```python
from build123d import *

# Parameters (mm, degrees)
CUT_EXTRUDE1_START = 7.29361
CUT_EXTRUDE1_DEPTH = 2.477670997


# Read off the part's stored shape, not the designer's step: Split1
with BuildPart() as part:
    # Sketch2 → Revolve1 (revolve)
    with BuildSketch(Plane(origin=(0, 0, 0), x_dir=(0, 0, -1), z_dir=(1, 0, 0)), mode=Mode.PRIVATE) as revolve1_sk:
        with BuildLine():
            Line((-7.89305, 0.79375), (-7.89305, 1.11125))
            ThreePointArc((-7.89305, 1.11125), (-7.36812089, 2.018629974), (-6.575878571, 2.7051))
            Line((-6.575878571, 2.7051), (-6.39445, 2.7051))
            Line((-6.39445, 2.7051), (-6.39445, 1.4224))
            Line((-6.39445, 1.4224), (7.4168, 1.4224))
            Line((7.4168, 1.4224), (7.89305, 0.94615))
            Line((7.89305, 0.94615), (7.89305, 0))
            Line((7.89305, 0), (-6.835338224, 0))
            Line((-6.835338224, 0), (-7.29361, 0.79375))
            Line((-7.29361, 0.79375), (-7.89305, 0.79375))
        make_face()
    revolve(revolve1_sk.sketch.rotate(Axis((0, 0, 7.89305), (0, 0, -1)), 90), axis=Axis((0, 0, 7.89305), (0, 0, -1)))

    # Sketch3 → Cut-Extrude1 (cut, through all)
    with BuildSketch(Plane.XY.offset(CUT_EXTRUDE1_START)):
        Polygon((0, 0.916543552), (-0.79375, 0.458271776), (-0.79375, -0.458271776), (0, -0.916543552), (0.79375, -0.458271776), (0.79375, 0.458271776), align=None)
    extrude(amount=CUT_EXTRUDE1_DEPTH, mode=Mode.SUBTRACT)

    # Cut-Extrude2 cone 1 section (through the dimple's axis) → Cut-Extrude2 (revolve, cut)
    with BuildSketch(Plane(origin=(0, 0, 7.89305), x_dir=(0, -1, 0), z_dir=(1, 0, 0))):
        Polygon((0, 0), (0.916543552, 0), (0, 0.916543552), align=None)
    revolve(axis=Axis((0, 0, 7.89305), (0, 0, -1)), mode=Mode.SUBTRACT)


with BuildPart() as body_2:
    # Split1: the piece on the far side of the plane
    add(part.part)
    split(bisect_by=Plane.XY.offset(6.39445), keep=Keep.BOTTOM)


with BuildPart() as part_1:
    add(part.part)

    # Split1
    split(bisect_by=Plane.XY.offset(6.39445), keep=Keep.TOP)

    add(body_2.part)  # Boss-Extrude1 merges body 2
    # Boss-Extrude1 cone 1 section (through the dimple's axis) → Boss-Extrude1 (revolve)
    with BuildSketch(Plane(origin=(0, 0, 6.39445), x_dir=(0, -1, 0), z_dir=(1, 0, 0))):
        Polygon((0, 0), (1.429512, 0), (0, 2.475987414), align=None)
    revolve(axis=Axis((0, 0, 6.39445), (0, 0, -1)))


solid = part_1.part
```
Geometry: final body of the model. Coordinates: model frame, mm. Round coordinates to 2 decimals unless told otherwise and drop trailing zeros. Order: outer loops, then holes, each group sorted by start corner. A loop starts at its lowest first (then second) coordinate and runs counter-clockwise, first axis right, second up. Notation, with made-up numbers: (-30.75, 74.5) - (26.25, 74.5) arc R30 cw to (26.25, 97.5) - close; hole circle Ø9 at (18, 32.25). An arc over 180 degrees is marked (long way). Use CSV: the item, a comma, the result in double quotes. Start each with the question number.
Q1. Mould query, pull axis X, two halves, no side actions, for faces 1 (the face through (0, 0, -7.893)), 2 (the face through (0.131, -0.041, 6.915)), 3 (the face through (0.66, 1.26, -0.61)). Classes: +X half, -X half, draft (parallel to the pull), parting line (faces both ways), or undercut.
Q2. Section query A-A (z = 4.5). Return loops of the section in (x, y), and give its area (3 significant figures).
Q3. First-contact query: pin 1 (2 mm diameter, centred on x = -1, z = 0, fed in from +Y); pin 2 (3 mm diameter, centred on x = 2, y = 2, fed in from -Z); pin 3 (0.7 mm diameter, centred on y = 0, z = 7.5, fed in from +X). Flat tips, straight axial feed; report the tip coordinate or a pass-through.
Q4. Section query B-B (y = 2.2). Return loops of the section in (x, z).
Q5. Material intervals for line 1 along Y through (x, z) = (0.95, -2); line 2 along Z through (x, y) = (-0.05, -1.35); line 3 along Y through (x, z) = (-0.05, 7), sorted ascending. Write a range as from..to.
Result set:
1,face 1,"draft"
1,face 2,"undercut"
1,face 3,"parting line"
2,outline,"circle Ø2.84 at (0, 0)"
2,area,"6.36 mm2"
3,pin 1,"stops at y = 1.42"
3,pin 2,"stops at z = -7.51"
3,pin 3,"stops at x = 2.26"
4,outline,"(-1.57, 6.39) - (1.57, 6.39) - (1.57, 6.58) arc R2.28 ccw to (-1.57, 6.58) - close"
5,line 1,"y = -1.06..1.06"
5,line 2,"z = -7.49..7.79"
5,line 3,"y = -2.39..-0.28, 0.28..2.39"
